from build123d import *

# Parameters (mm, degrees)
BASES_W                              = 17.8
BASES_H                              = 25.7
BASE_DEPTH                           = 1.5
NEUTRALS_W                           = 1.3
NEUTRALS_H                           = 7.3
NEUTRAL_DEPTH                        = 1.6
FASTENERACCESSS_R                    = 4
FASTENER_ACCESS_DEPTH                = 1
GROUNDS_W                            = 7.3
GROUNDS_H                            = 1.3
GROUND_DEPTH                         = 1.6
BASETOPS_W                           = 17.8
BASETOPS_H                           = 1.5
BASE_TOP_DEPTH                       = 14.5
BASERIGHTWALLS_W                     = 1.5
BASERIGHTWALLS_H                     = 10.2
BASE_RIGHT_WALL_DEPTH                = 14.5
CONNECTORWALLS_W                     = 1.8
CONNECTORWALLS_H                     = 10.2
CONNECTOR_WALL_DEPTH                 = 14.5
CONNECTOR_LOCATE_REACH               = 33.555
CONNECTORLOCATES_W                   = 3.9
CONNECTORLOCATES_H                   = 4
BASEBOTTOMS_W                        = 17.8
BASEBOTTOMS_H                        = 2
BASE_BOTTOM_DEPTH                    = 14.5
FASTENERACCESSHOLEEXTENDS_R          = 2.75
FASTENER_ACCESS_HOLE_EXTEND_DEPTH    = 22.664083179
FASTENER_HOLDING_BODY_DEPTH          = 14.5
FASTENERHOLDINGTOPBORES_R            = 2.75
FASTENER_HOLDING_TOP_BORE_DEPTH      = 8.1
FASTENERHOLDINGBORES_R               = 1.75
FASTENER_HOLDING_BORE_DEPTH          = 19.343731899
ELECTRICALCONNECTIONBASES_W          = 3.9
ELECTRICALCONNECTIONBASES_H          = 1
ELECTRICAL_CONNECTION_BASE_DEPTH     = 14.5
CONNECTIONS_MIDWALL_JOINT_DEPTH      = 14.5
FASTENERHOLDINGEXTENDEDBODYS_R       = 2.5
FASTENERHOLDINGEXTENDEDBODYS_R_2     = 1.75
FASTENER_HOLDING_EXTENDED_BODY_DEPTH = 8.8
FHEB_SLOT_REACH                      = 31.315
FHEB_SLOT_DIRECTION_2_REACH          = 31.315
MIDWALLENDS_W                        = 2.2
MIDWALLENDS_H                        = 1.527350455
MID_WALL_END_DEPTH                   = 14.5
GROUNDWALLS_W                        = 1.5
GROUNDWALLS_H                        = 6
GROUND_WALL_DEPTH                    = 14.5
GROUNDEXTENDEDWALLSS_W               = 10.05
GROUNDEXTENDEDWALLSS_H               = 2
GROUNDEXTENDEDWALLSS_W_2             = 1.5
GROUNDEXTENDEDWALLSS_H_2             = 1.5
GROUND_EXTENDED_WALLS_DEPTH          = 14.5
GROUNDENDWALLS_W                     = 0.85
GROUNDENDWALLS_H                     = 3.5
GROUND_END_WALL_DEPTH                = 14.5
GROUND_CONNECTOR_LOCATE_REACH        = 34.595
GROUNDCONNECTORLOCATES_W             = 4
GROUNDCONNECTORLOCATES_H             = 4


# Read off the part's stored shape, not the designer's step: FHEB DRAFT
with BuildPart() as part:
    # BaseS → BASE (new body)
    with BuildSketch(Plane.XY):
        Rectangle(BASES_W, BASES_H)
    extrude(amount=-BASE_DEPTH)

    # NeutralS → NEUTRAL (cut)
    with BuildSketch(Plane.XY):
        with Locations((5.45, 5.8)):
            Rectangle(NEUTRALS_W, NEUTRALS_H)
    neutral = extrude(amount=-NEUTRAL_DEPTH, mode=Mode.SUBTRACT)

    # LINE HM: NEUTRAL across plane
    add(neutral.mirror(Plane(origin=(0, 0, 0), x_dir=(0, 0, 1), z_dir=(1, 0, 0))), mode=Mode.SUBTRACT)

    # FastenerAccessS → FASTENER ACCESS (cut)
    with BuildSketch(Plane.XY):
        Circle(FASTENERACCESSS_R)
    extrude(amount=-FASTENER_ACCESS_DEPTH, mode=Mode.SUBTRACT)

    # GroundS → GROUND (cut)
    with BuildSketch(Plane.XY):
        with Locations((0, -8.7)):
            Rectangle(GROUNDS_W, GROUNDS_H)
    extrude(amount=-GROUND_DEPTH, mode=Mode.SUBTRACT)

    # BaseTopS → BASE TOP (add)
    with BuildSketch(Plane(origin=(0, 0, -1.5), x_dir=(-1, 0, 0), z_dir=(0, 0, -1))):
        with Locations((0, 12.1)):
            Rectangle(BASETOPS_W, BASETOPS_H)
    extrude(amount=BASE_TOP_DEPTH)

    # BaseRightWallS → BASE RIGHT WALL (add)
    with BuildSketch(Plane(origin=(0, 0, -1.5), x_dir=(-1, 0, 0), z_dir=(0, 0, -1))):
        with Locations((-8.15, 6.25)):
            Rectangle(BASERIGHTWALLS_W, BASERIGHTWALLS_H)
    base_right_wall = extrude(amount=BASE_RIGHT_WALL_DEPTH)

    # ConnectorWallS → CONNECTOR WALL (add)
    with BuildSketch(Plane(origin=(0, 0, -1.5), x_dir=(-1, 0, 0), z_dir=(0, 0, -1))):
        with Locations((-2.6, 6.25)):
            Rectangle(CONNECTORWALLS_W, CONNECTORWALLS_H)
    connector_wall = extrude(amount=CONNECTOR_WALL_DEPTH)

    # ConnectorLocateS → CONNECTOR LOCATE (cut, up to next)
    with BuildSketch(Plane(origin=(0, 12.85, 0), x_dir=(-1, 0, 0), z_dir=(0, 1, 0)), mode=Mode.PRIVATE) as connector_locate_sk1:
        with Locations((-5.45, -14)):
            Rectangle(CONNECTORLOCATES_W, CONNECTORLOCATES_H)
    connector_locate_tool1 = extrude(connector_locate_sk1.sketch, amount=-CONNECTOR_LOCATE_REACH, mode=Mode.PRIVATE) & part.part
    connector_locate = connector_locate_tool1.solids().sort_by_distance((5.45, 12.85, -14))[0]
    add(connector_locate, mode=Mode.SUBTRACT)

    # CW CL HM: BASE RIGHT WALL, CONNECTOR WALL, CONNECTOR LOCATE across plane
    add(base_right_wall.mirror(Plane(origin=(0, 0, 0), x_dir=(0, 0, 1), z_dir=(1, 0, 0))))
    add(connector_wall.mirror(Plane(origin=(0, 0, 0), x_dir=(0, 0, 1), z_dir=(1, 0, 0))))
    add(connector_locate.mirror(Plane(origin=(0, 0, 0), x_dir=(0, 0, 1), z_dir=(1, 0, 0))), mode=Mode.SUBTRACT)

    # BaseBottomS → BASE BOTTOM (add)
    with BuildSketch(Plane(origin=(0, 0, -1.5), x_dir=(-1, 0, 0), z_dir=(0, 0, -1))):
        with Locations((0, -11.85)):
            Rectangle(BASEBOTTOMS_W, BASEBOTTOMS_H)
    extrude(amount=BASE_BOTTOM_DEPTH)

    # FastenerAccessHoleExtendS → FASTENER ACCESS HOLE EXTEND (cut, through all)
    with BuildSketch(Plane.XY.offset(-1)):
        Circle(FASTENERACCESSHOLEEXTENDS_R)
    extrude(amount=-FASTENER_ACCESS_HOLE_EXTEND_DEPTH, mode=Mode.SUBTRACT)

    # FastenerHoldingBodyS → FASTENER HOLDING BODY (add)
    with BuildSketch(Plane(origin=(0, 0, -1.5), x_dir=(-1, 0, 0), z_dir=(0, 0, -1))):
        with BuildLine():
            Line((-3.5, 0), (-3.5, 1.15))
            Line((-3.5, 1.15), (-3.305676935, 1.15))
            ThreePointArc((-3.305676935, 1.15), (0, 3.5), (3.305676935, 1.15))
            Line((3.305676935, 1.15), (3.5, 1.15))
            Line((3.5, 1.15), (3.5, 0))
            ThreePointArc((3.5, 0), (0, -3.5), (-3.5, 0))
        make_face()
    extrude(amount=FASTENER_HOLDING_BODY_DEPTH)

    # FastenerHoldingTopBoreS → FASTENER HOLDING TOP BORE (cut)
    with BuildSketch(Plane.XY.offset(-1.5)):
        Circle(FASTENERHOLDINGTOPBORES_R)
    extrude(amount=-FASTENER_HOLDING_TOP_BORE_DEPTH, mode=Mode.SUBTRACT)

    # FastenerHoldingBoreS → FASTENER HOLDING BORE (cut, through all)
    with BuildSketch(Plane.XY.offset(-9.6)):
        Circle(FASTENERHOLDINGBORES_R)
    extrude(amount=-FASTENER_HOLDING_BORE_DEPTH, mode=Mode.SUBTRACT)

    # ElectricalConnectionBaseS → ELECTRICAL CONNECTION BASE (add)
    with BuildSketch(Plane(origin=(0, 0, -1.5), x_dir=(-1, 0, 0), z_dir=(0, 0, -1))):
        with Locations((-5.45, 1.65)):
            Rectangle(ELECTRICALCONNECTIONBASES_W, ELECTRICALCONNECTIONBASES_H)
        with Locations((5.45, 1.65)):
            Rectangle(ELECTRICALCONNECTIONBASES_W, ELECTRICALCONNECTIONBASES_H)
    extrude(amount=ELECTRICAL_CONNECTION_BASE_DEPTH)

    # ConnectionsMidwallJointS → CONNECTIONS MIDWALL JOINT (add)
    with BuildSketch(Plane(origin=(0, 0, -1.5), x_dir=(-1, 0, 0), z_dir=(0, 0, -1))):
        with BuildLine():
            Line((-1.7, 3.95), (1.7, 3.95))
            Line((1.7, 3.95), (1.7, 3.059411708))
            ThreePointArc((1.7, 3.059411708), (0, 3.5), (-1.7, 3.059411708))
            Line((-1.7, 3.059411708), (-1.7, 3.95))
        make_face()
    extrude(amount=CONNECTIONS_MIDWALL_JOINT_DEPTH)

    # FastenerHoldingExtendedBodyS → FASTENER HOLDING EXTENDED BODY (add)
    with BuildSketch(Plane(origin=(0, 0, -16), x_dir=(-1, 0, 0), z_dir=(0, 0, -1))):
        with Locations(Location((0, 0, 0), (0, 0, 180))):
            Circle(FASTENERHOLDINGEXTENDEDBODYS_R)
        with Locations(Location((0, 0, 0), (0, 0, 180))):
            Circle(FASTENERHOLDINGEXTENDEDBODYS_R_2, mode=Mode.SUBTRACT)
    extrude(amount=FASTENER_HOLDING_EXTENDED_BODY_DEPTH)

    # FHEBSlotS → FHEB SLOT (cut, up to next)
    with BuildSketch(Plane(origin=(0, 0, 0), x_dir=(0, 0, -1), z_dir=(1, 0, 0)), mode=Mode.PRIVATE) as fheb_slot_sk1:
        with BuildLine():
            Line((24.8, -0.35), (19.8, -0.35))
            ThreePointArc((19.8, -0.35), (19.45, 0), (19.8, 0.35))
            Line((19.8, 0.35), (24.8, 0.35))
            Line((24.8, 0.35), (24.8, -0.35))
        make_face()
    fheb_slot_tool1 = extrude(fheb_slot_sk1.sketch, amount=-FHEB_SLOT_REACH, mode=Mode.PRIVATE) & part.part
    add(fheb_slot_tool1.solids().sort_by_distance((0, 0, -22.161977))[0], mode=Mode.SUBTRACT)

    # FHEBSlotS → FHEB SLOT direction 2 (cut, up to next)
    with BuildSketch(Plane(origin=(0, 0, 0), x_dir=(0, 0, -1), z_dir=(1, 0, 0)), mode=Mode.PRIVATE) as fheb_slot_direction_2_sk1:
        with BuildLine():
            Line((24.8, -0.35), (19.8, -0.35))
            ThreePointArc((19.8, -0.35), (19.45, 0), (19.8, 0.35))
            Line((19.8, 0.35), (24.8, 0.35))
            Line((24.8, 0.35), (24.8, -0.35))
        make_face()
    fheb_slot_direction_2_tool1 = extrude(fheb_slot_direction_2_sk1.sketch, amount=FHEB_SLOT_DIRECTION_2_REACH, mode=Mode.PRIVATE) & part.part
    add(fheb_slot_direction_2_tool1.solids().sort_by_distance((0, 0, -22.161977))[0], mode=Mode.SUBTRACT)

    # MidWallEndS → MID WALL END (add)
    with BuildSketch(Plane(origin=(0, 0, -1.5), x_dir=(-1, 0, 0), z_dir=(0, 0, -1))):
        with Locations((0, -4.086324773)):
            Rectangle(MIDWALLENDS_W, MIDWALLENDS_H)
    extrude(amount=MID_WALL_END_DEPTH)

    # GroundWallS → GROUND WALL (add)
    with BuildSketch(Plane(origin=(0, 0, -1.5), x_dir=(-1, 0, 0), z_dir=(0, 0, -1))):
        with Locations((-7.15, -7.85)):
            Rectangle(GROUNDWALLS_W, GROUNDWALLS_H)
    extrude(amount=GROUND_WALL_DEPTH)

    # GroundExtendedWallsS → GROUND EXTENDED WALLS (add)
    with BuildSketch(Plane(origin=(0, 0, -1.5), x_dir=(-1, 0, 0), z_dir=(0, 0, -1))):
        with Locations((-1.375, -5.85)):
            Rectangle(GROUNDEXTENDEDWALLSS_W, GROUNDEXTENDEDWALLSS_H)
        with Locations((2.9, -10.1)):
            Rectangle(GROUNDEXTENDEDWALLSS_W_2, GROUNDEXTENDEDWALLSS_H_2)
    extrude(amount=GROUND_EXTENDED_WALLS_DEPTH)

    # GroundEndWallS → GROUND END WALL (add)
    with BuildSketch(Plane(origin=(0, 0, -1.5), x_dir=(-1, 0, 0), z_dir=(0, 0, -1))):
        with Locations((4.075, -8.1)):
            Rectangle(GROUNDENDWALLS_W, GROUNDENDWALLS_H)
    extrude(amount=GROUND_END_WALL_DEPTH)

    # FHEB DRAFT outline → FHEB DRAFT (revolve, cut)
    with BuildSketch(Plane.XZ):
        Polygon((2.5, -16), (2.346395429, -24.8), (2.5, -24.8), align=None)
    revolve(axis=Axis((0, 0, 0), (0, 0, 1)), mode=Mode.SUBTRACT)

    # GroundConnectorLocateS → GROUND CONNECTOR LOCATE (cut, up to next)
    with BuildSketch(Plane(origin=(7.9, 0, 0), x_dir=(0, 0, -1), z_dir=(1, 0, 0)), mode=Mode.PRIVATE) as ground_connector_locate_sk1:
        with Locations((14, -8.85)):
            Rectangle(GROUNDCONNECTORLOCATES_W, GROUNDCONNECTORLOCATES_H)
    ground_connector_locate_tool1 = extrude(ground_connector_locate_sk1.sketch, amount=-GROUND_CONNECTOR_LOCATE_REACH, mode=Mode.PRIVATE) & part.part
    add(ground_connector_locate_tool1.solids().sort_by_distance((7.9, -8.85, -14))[0], mode=Mode.SUBTRACT)


solid = part.part
Here's how the part is built. I have some questions about the finished solid (model axes, mm). A direction names the side the tool comes from. Coordinates: 2 decimals unless noted, no trailing zeros. Write each loop counter-clockwise with the first axis right and the second up, starting at its lowest first coordinate (ties: lowest second). Pieces come first, ordered by that corner, then holes.
Item 1: I want a section at C-C on x = 0. Count the separate pieces of the cut face and the enclosed holes in it, and give its area (3 significant figures).
Item 2: I want a section at A-A on y = 7.25. Write out the boundary of the cut face in (x, z).
Item 3: Will these pins go through, and if not, where does the flat tip stop? pin 1 (8 mm diameter, centred on x = -3, y = -1.5, fed in from +Z); pin 2 (4 mm diameter, centred on x = -4.5, y = 6, fed in from -Z); pin 3 (1.5 mm diameter, centred on y = -3, z = -10, fed in from -X); pin 4 (0.8 mm diameter, centred on y = -8.5, z = -8.5, fed in from +X).
Item 4: On a 3-axis mill with a long thin cutter (end or side, diameter ignored), from which of +Z, -Z, +X, -X, +Y, -Y can I reach the whole of each face in a straight line? I mean faces 1 (the flat face through (-4, -6.35, -9)), 2 (the flat face through (-6.1, 6, -1)), 3 (the flat face through (-2.15, -10, -9)). Say none if no direction works.
Item 5: I want a section at B-B on y = 10. Write out the boundary of the cut face in (x, z).
Item 6: If I drill on line 1 (Y direction, x = 6.75, z = -15.5); line 2 (X direction, y = 5.25, z = -2); line 3 (Y direction, x = -5.5, z = -10.5), over which ranges is the centre line in solid material (lowest first)?
Item 7: If we mould it in two halves opening along X, with no side actions, what happens to faces 4 (the flat face through (-1.1, -4, -9)), 5 (the flat face through (0, 8, -1.5)), 6 (the flat face through (0, 2, -24.8))? For each: +X half, -X half, draft (parallel to the pull), parting line (faces both ways), or undercut.
Findings below:
1. separate pieces: 3
1. enclosed holes: 0
1. area: 178 mm2
2. outline: (-8.9, -16) - (-7.4, -16) - (-7.4, -1.5) - (-6.1, -1.5) - (-6.1, 0) - (-8.9, 0) - close; (-4.8, -1.5) - (-3.5, -1.5) - (-3.5, -16) - (-1.7, -16) - (-1.7, -1.5) - (1.7, -1.5) - (1.7, -16) - (3.5, -16) - (3.5, -1.5) - (4.8, -1.5) - (4.8, 0) - (-4.8, 0) - close; (6.1, -1.5) - (7.4, -1.5) - (7.4, -16) - (8.9, -16) - (8.9, 0) - (6.1, 0) - close
3. pin 1: stops at z = 0
3. pin 2: stops at z = -16
3. pin 3: stops at x = -2.68
3. pin 4: stops at x = 7.9
4. face 1: -Z, -X
4. face 2: +Z, -Z
4. face 3: -Z
5. outline: (-8.9, -16) - (-7.4, -16) - (-7.4, -1.5) - (-3.5, -1.5) - (-3.5, -16) - (-1.7, -16) - (-1.7, -1.5) - (1.7, -1.5) - (1.7, -16) - (3.5, -16) - (3.5, -1.5) - (7.4, -1.5) - (7.4, -16) - (8.9, -16) - (8.9, 0) - (-8.9, 0) - close
6. line 1: y = -12.85 to -10.85, -6.85 to -4.85, 1.15 to 2.15
6. line 2: x = -8.9 to -7.4, -3.5 to -1.7, 1.7 to 3.5, 7.4 to 8.9
6. line 3: y = -12.85 to -10.85, 1.15 to 2.15, 11.35 to 12.85
7. face 4: -X half
7. face 5: undercut
7. face 6: draft
